Design review of the part shown in the three views and the two pictorial views. Dimensions are in mm from the part's minimum x, y and z. Give positions to 0.01 mm unless a question says otherwise; leave off trailing zeros. Loops run counter-clockwise (first coordinate to the right, second up) from the corner with the lowest first, then second, coordinate; pieces in that order, holes last. Notation, with made-up numbers: (-31.5, 75.25) -> (-6.5, 75.25) arc R10 cw to (-6.5, 92.25) -> close; hole circle Ø4 at (44, -11.5). An arc over 180 degrees is marked (long way). Answer as CSV lines item,"result".
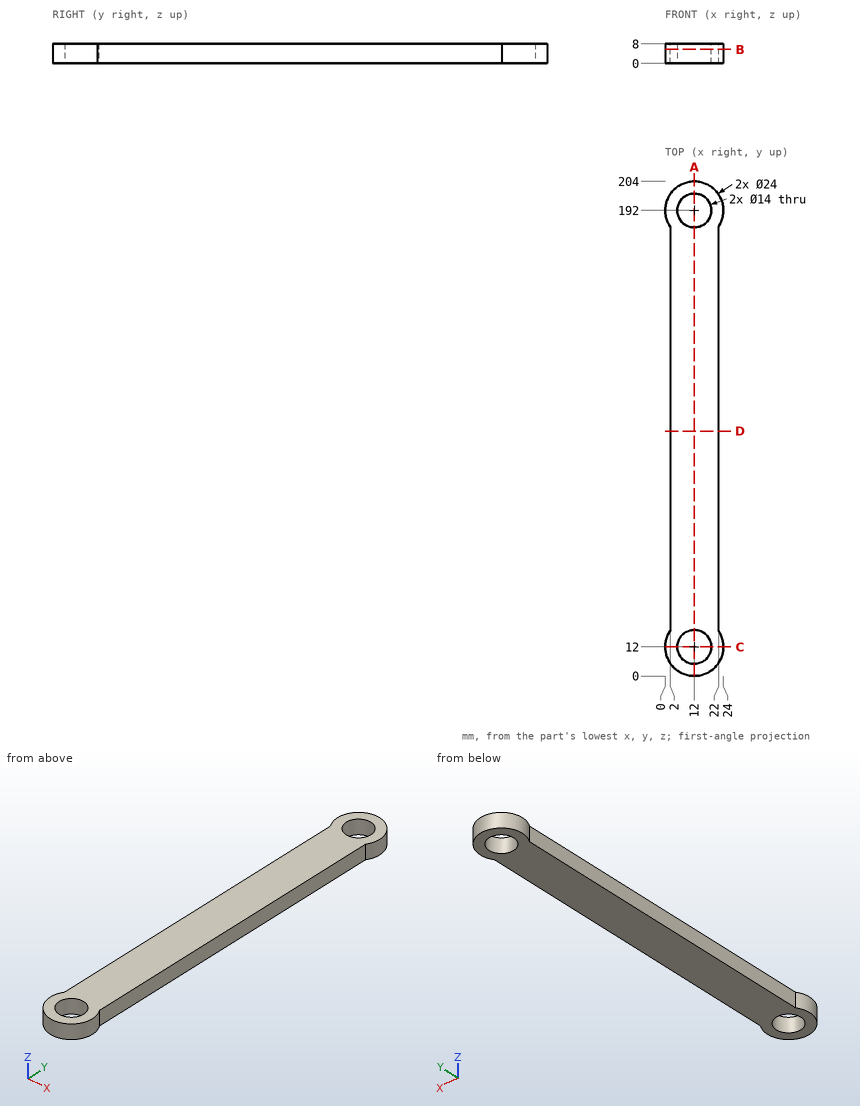
Q1. We need section C-C, the plane y = 12. State the section outline as (x, z) points, and give its area (3 significant figures).
Filled sheet:
outline,"(0, 0) -> (5, 0) -> (5, 8) -> (0, 8) -> close; (19, 0) -> (24, 0) -> (24, 8) -> (19, 8) -> close"
area,"80.0 mm^2"
Q2. Clearance check with flat-ended pins moving along their axes: pin 1 Ø2.5 at (y, z) = (71.5, 3.5) entering from -X; pin 2 Ø2 at (x, z) = (4.5, 6) entering from -Y. State where each tip first meets the part, or that it passes through.
Filled sheet:
pin 1,"stops at x = 2"
pin 2,"stops at y = 1.91"
Q3. We need section B-B, the plane z = 5.75. State the section outline as (x, y) points, and give its area (3 significant figures).
Filled sheet:
outline,"(2, 18.63) arc R12 ccw (long way) to (22, 18.63) -> (22, 185.37) arc R12 ccw (long way) to (2, 185.37) -> close; hole circle Ø14 at (12, 12); hole circle Ø14 at (12, 192)"
area,"3,780 mm^2"
Q4. We need section D-D, the plane y = 101. State the section outline as (x, z) points, and give its area (3 significant figures).
Filled sheet:
outline,"(2, 0) -> (22, 0) -> (22, 8) -> (2, 8) -> close"
area,"160 mm^2"
Q5. We need section A-A, the plane x = 12. State the section outline as (y, z) points, and give its area (3 significant figures).
Filled sheet:
outline,"(0, 0) -> (5, 0) -> (5, 8) -> (0, 8) -> close; (19, 0) -> (185, 0) -> (185, 8) -> (19, 8) -> close; (199, 0) -> (204, 0) -> (204, 8) -> (199, 8) -> close"
area,"1,410 mm^2"
Q6. To check wall thickness, follow probe 1 along Y at (x, z) = (12, 5.75); probe 2 along X at (y, z) = (192, 2); probe 3 along Y at (x, z) = (14.25, 0.5). State the ranges of each line that lie inside material, in increasing order. Write a range as from..to.
Filled sheet:
probe 1,"y = 0..5, 19..185, 199..204"
probe 2,"x = 0..5, 19..24"
probe 3,"y = 0.21..5.37, 18.63..185.37, 198.63..203.79"
